```python
from build123d import *

# Parameters (mm, degrees)
BOSS_EXTRUDE1_DEPTH = 1.524


with BuildPart() as part:
    # Sketch1 → Boss-Extrude1 (new body)
    with BuildSketch(Plane.XY):
        with BuildLine():
            Line((12.801369516, 0), (12.801369516, -1.524))
            Line((12.801369516, -1.524), (10.391932007, -1.524))
            ThreePointArc((10.391932007, -1.524), (10.729282299, -3.576784737), (12.438012127, -4.763365021))
            ThreePointArc((12.438012127, -4.763365021), (17.707377285, -5.836214945), (22.697391826, -3.831976686))
            ThreePointArc((22.697391826, -3.831976686), (24.001804643, -5.463328455), (26.08664711, -5.335918573))
            ThreePointArc((26.08664711, -5.335918573), (28.593778041, -4.308492819), (31.181851225, -3.506503807))
            Line((31.181851225, -3.506503807), (32.184006456, -5.335918573))
            Line((32.184006456, -5.335918573), (32.373708357, -3.219533349))
            ThreePointArc((32.373708357, -3.219533349), (34.925372654, -2.771007765), (37.505800807, -2.53958514))
            Line((37.505800807, -2.53958514), (38.45795608, -4.277725961))
            Line((38.45795608, -4.277725961), (38.950884125, -2.505498906))
            ThreePointArc((38.950884125, -2.505498906), (41.098053648, -2.580802933), (43.234672107, -2.806344974))
            Line((43.234672107, -2.806344974), (43.234672107, -4.277725961))
            Line((43.234672107, -4.277725961), (44.101614036, -2.941400649))
            ThreePointArc((44.101614036, -2.941400649), (47.285508928, -3.660506996), (50.374872797, -4.714134778))
            Line((50.374872797, -4.714134778), (50.374872797, -6.206057494))
            Line((50.374872797, -6.206057494), (51.106289172, -5.018968989))
            ThreePointArc((51.106289172, -5.018968989), (54.742715091, -6.887018604), (58.098173874, -9.222419893))
            ThreePointArc((58.098173874, -9.222419893), (60.731696449, -9.312826177), (61.868627066, -6.935642292))
            ThreePointArc((61.868627066, -6.935642292), (61.317201318, -5.297304696), (60.822209833, -3.641042681))
            Line((60.822209833, -3.641042681), (61.432885238, -2.890340871))
            Line((61.432885238, -2.890340871), (60.618018518, -2.890340871))
            ThreePointArc((60.618018518, -2.890340871), (59.887453188, 0.294487754), (59.364520303, 3.519918))
            Line((59.364520303, 3.519918), (59.938762272, 4.044130938))
            Line((59.938762272, 4.044130938), (59.292703769, 4.103102621))
            ThreePointArc((59.292703769, 4.103102621), (59.05887021, 6.657377407), (58.95511856, 9.220233903))
            Line((58.95511856, 9.220233903), (59.938762272, 9.426656134))
            Line((59.938762272, 9.426656134), (58.949679492, 9.813602305))
            ThreePointArc((58.949679492, 9.813602305), (59.020268562, 12.652910586), (59.250476195, 15.483751235))
            Line((59.250476195, 15.483751235), (60.304285386, 15.979807686))
            Line((60.304285386, 15.979807686), (59.371854232, 16.495625036))
            ThreePointArc((59.371854232, 16.495625036), (59.625803461, 18.214330904), (59.938762272, 19.923277028))
            ThreePointArc((59.938762272, 19.923277028), (60.072497403, 20.30995458), (60.304285386, 20.647117664))
            ThreePointArc((60.304285386, 20.647117664), (61.605742963, 23.863190011), (60.513628087, 27.156243043))
            ThreePointArc((60.513628087, 27.156243043), (60.316413067, 27.479275668), (60.204881845, 27.840944893))
            ThreePointArc((60.204881845, 27.840944893), (59.887129724, 30.355756102), (59.816689824, 32.889583256))
            Line((59.816689824, 32.889583256), (60.618018518, 33.060793415))
            Line((60.618018518, 33.060793415), (59.835472852, 33.469819147))
            ThreePointArc((59.835472852, 33.469819147), (60.265577513, 37.173766341), (61.223023534, 40.77758542))
            Line((61.223023534, 40.77758542), (61.868627066, 40.77758542))
            Line((61.868627066, 40.77758542), (61.345913077, 41.12626446))
            ThreePointArc((61.345913077, 41.12626446), (63.032929734, 44.85342804), (65.285725915, 48.268495084))
            Line((65.285725915, 48.268495084), (66.32927785, 47.988149788))
            Line((66.32927785, 47.988149788), (65.763533096, 48.863100705))
            ThreePointArc((65.763533096, 48.863100705), (69.158811096, 52.264251778), (73.1239346, 54.979677512))
            Line((73.1239346, 54.979677512), (73.693442296, 54.520997073))
            Line((73.693442296, 54.520997073), (73.693442296, 55.287173458))
            ThreePointArc((73.693442296, 55.287173458), (75.566961014, 56.175053965), (77.50548515, 56.910260303))
            Line((77.50548515, 56.910260303), (75.543932889, 56.910260303))
            ThreePointArc((75.543932889, 56.910260303), (60.978808558, 45.393240793), (57.46632066, 27.160111223))
            ThreePointArc((57.46632066, 27.160111223), (57.643802358, 26.659339703), (57.982404007, 26.24992452))
            ThreePointArc((57.982404007, 26.24992452), (59.006767547, 24.18711185), (58.217688211, 22.023348792))
            ThreePointArc((58.217688211, 22.023348792), (57.974404382, 21.680039515), (57.834272182, 21.283288652))
            ThreePointArc((57.834272182, 21.283288652), (56.763038041, 7.682552112), (59.02088406, -5.772175992))
            ThreePointArc((59.02088406, -5.772175992), (58.884555424, -6.959716199), (57.933337254, -7.683609307))
            ThreePointArc((57.933337254, -7.683609307), (42.379716063, 0.214147761), (24.937129111, 0))
            ThreePointArc((24.937129111, 0), (22.427681087, 5.112001973), (16.861199629, 6.313741433))
            ThreePointArc((16.861199629, 6.313741433), (12.668346736, 4.819065663), (10.729282299, 0.812308851))
            Line((10.729282299, 0.812308851), (10.729282299, 0))
            Line((10.729282299, 0), (12.801369516, 0))
        make_face()
    extrude(amount=BOSS_EXTRUDE1_DEPTH)


solid = part.part
```
Geometry: final body of the model. Coordinates: model frame, mm. A direction names the side the tool comes from. Coordinates: 2 decimals unless noted, no trailing zeros. Order: outer loops, then holes, each group sorted by start corner. A loop starts at its lowest first (then second) coordinate and runs counter-clockwise, first axis right, second up.
Item 1: Section query B-B (x = 20). Output: boundary loops of the cut face in (y, z), then the cut area to 3 significant figures.
Answer:
outline: (-5.33, 0) - (6.3, 0) - (6.3, 1.52) - (-5.33, 1.52) - close
area: 17.7 mm2
Item 2: Access query for faces 1 (the face through (32.278, -4.293, 0.751)), 2 (the face through (12, -1.524, 1)), 3 (the face through (59.62, 18.19, 0.75)), 4 (the face through (77, 56.91, 1)). Directions: +Z, -Z, +X, -X, +Y, -Y. A direction counts if a zero-diameter tool reaches every point of the face in a straight line with its end or side. Return the directions, or none.
Answer:
face 1: +Z, -Z, -Y
face 2: +Z, -Z, -X
face 3: +Z, -Z, +X
face 4: +Z, -Z, +X, -X, +Y
Item 3: Material intervals for line 1 along X through (y, z) = (10.5, 0.1); line 2 along X through (y, z) = (-2, 0.8); line 3 along X through (y, z) = (24, 1.4), sorted ascending.
Answer:
line 1: x = 56.71 to 58.95
line 2: x = 10.32 to 48.97, 58.04 to 60.39
line 3: x = 59.01 to 61.61
Item 4: Section query A-A (y = 35). Output: boundary loops of the cut face in (x, z), then the cut area to 3 significant figures.
Answer:
outline: (57.33, 0) - (59.95, 0) - (59.95, 1.52) - (57.33, 1.52) - close
area: 3.99 mm2
Item 5: Contact query for flat-ended pins moving along their axis: P1, Ø3, axis at x = 55, y = 5.5, coming from the -Z side; P2, Ø0.7, axis at x = 61.5, z = 1, coming from the -Y side; P3, Ø0.5, axis at x = 11, z = 1, coming from the +Y side; P4, Ø0.6, axis at y = 0.5, z = 0.5, coming from the -X side. Output: stop coordinate, or through.
Answer:
P1: passes through
P2: stops at y = -8.99
P3: stops at y = 2.89
P4: stops at x = 10.73
Item 6: Draft query along X for faces 5 (the face through (56.755, 7.874, 0.751)), 6 (the face through (41, -1, 0)), 7 (the face through (10.713, -3.551, 0.751)), 8 (the face through (59.896, 0.25, 0.751)). Return one class per face: released by +X, released by -X, zero draft, split by the parting line, or undercut.
Answer:
face 5: undercut
face 6: zero draft
face 7: released by -X
face 8: released by +X
